```python
from build123d import *

# Parameters (mm, degrees)
SKETCH1_W           = 10
SKETCH1_H           = 10
BOSS_EXTRUDE1_DEPTH = 10
SKETCH2_R           = 2.5
BOSS_EXTRUDE2_DEPTH = 5
SKETCH3_R           = 1
CUT_EXTRUDE1_DEPTH  = 10
SKETCH4_R           = 0.5
CUT_EXTRUDE2_DEPTH  = 5


with BuildPart() as part:
    # Sketch1 → Boss-Extrude1 (new body)
    with BuildSketch(Plane(origin=(0, 0, 0), x_dir=(1, 0, 0), z_dir=(0, 1, 0))):
        with Locations((-9.64819331, 21.790774606)):
            Rectangle(SKETCH1_W, SKETCH1_H)
    extrude(amount=BOSS_EXTRUDE1_DEPTH)

    # Sketch2 → Boss-Extrude2 (add)
    with BuildSketch(Plane(origin=(0, 10, 0), x_dir=(1, 0, 0), z_dir=(0, 1, 0))):
        with Locations((-9.64819331, 21.790774606)):
            Circle(SKETCH2_R)
    extrude(amount=BOSS_EXTRUDE2_DEPTH)

    # Sketch3 → Cut-Extrude1 (cut)
    with BuildSketch(Plane.ZY.offset(14.64819331)):
        with Locations((-21.790774606, 5)):
            Circle(SKETCH3_R)
    extrude(amount=-CUT_EXTRUDE1_DEPTH, mode=Mode.SUBTRACT)

    # Sketch4 → Cut-Extrude2 (cut)
    with BuildSketch(Plane(origin=(0, 0, 0), x_dir=(-1, 0, 0), z_dir=(0, -1, 0))):
        with Locations((9.64819331, 21.790774606)):
            Circle(SKETCH4_R)
    extrude(amount=-CUT_EXTRUDE2_DEPTH, mode=Mode.SUBTRACT)


solid = part.part
```
For this review, take the finished solid that the model builds, in its own axes (mm). A direction names the side the tool comes from. Give positions to 0.01 mm unless a question says otherwise; leave off trailing zeros. Write each loop counter-clockwise with the first axis right and the second up, starting at its lowest first coordinate (ties: lowest second). Pieces come first, ordered by that corner, then holes.
Item 1: Take a section at A-A (x = -6.5). Give the boundary of the cut face in (y, z), and give its area (3 significant figures).
Item 2: Take a section at D-D (z = -23.75). Give the boundary of the cut face in (x, y).
Item 3: Take a section at C-C (z = -22). Give the boundary of the cut face in (x, y).
Item 4: The part is to be moulded in two halves that separate along Z. For faces 3 (the face through (-14.648, 5, -23)), 4 (the face through (-10, 5, -16.791)), 5 (the face through (-9.92, 2.04, -22.21)), say which applies: +Z half, -Z half, draft (parallel to the pull), parting line (faces both ways), or undercut.
Item 5: Wall thickness on probe 1 along Y at (x, z) = (-13.75, -18.25); probe 2 along Y at (x, z) = (-13.5, -21.25); probe 3 along Y at (x, z) = (-12.25, -21.75): over which ranges is each line inside the solid? List them lowest first.
Item 6: Take a section at B-B (y = 5). Give the boundary of the cut face in (x, z).
Item 7: Machinability: for faces 1 (the face through (-11, 0, -22)), 2 (the face through (-11.63, 12.46, -20.27)), which of the approach directions +Z, -Z, +X, -X, +Y, -Y give a long, thin tool a straight path to every point of the face, cutting with its end or side? Answer none if there is none.
Established:
1. outline: (0, -26.79) - (10, -26.79) - (10, -16.79) - (0, -16.79) - close; hole circle Ø2 at (5, -21.79)
1. area: 96.9 mm2
2. outline: (-14.65, 0) - (-4.65, 0) - (-4.65, 10) - (-8.1, 10) - (-8.1, 15) - (-11.2, 15) - (-11.2, 10) - (-14.65, 10) - close
3. outline: (-14.65, 0) - (-10.1, 0) - (-10.1, 4.02) - (-14.65, 4.02) - close; (-14.65, 5.98) - (-4.65, 5.98) - (-4.65, 10) - (-7.16, 10) - (-7.16, 15) - (-12.14, 15) - (-12.14, 10) - (-14.65, 10) - close; (-9.19, 0) - (-4.65, 0) - (-4.65, 4.02) - (-9.19, 4.02) - close
4. face 3: draft
4. face 4: +Z half
4. face 5: undercut
5. probe 1: y = 0 to 10
5. probe 2: y = 0 to 4.16, 5.84 to 10
5. probe 3: y = 0 to 4, 6 to 10
6. outline: (-14.65, -26.79) - (-4.65, -26.79) - (-4.65, -22.79) - (-14.65, -22.79) - close; (-14.65, -20.79) - (-4.65, -20.79) - (-4.65, -16.79) - (-14.65, -16.79) - close
7. face 1: +Z, -Z, +X, -X, -Y
7. face 2: +Y
